Check sheet for the modelled part. Datum: model origin and axes. Units: mm. A direction names the side the tool comes from. Give positions to 0.01 mm unless a question says otherwise; leave off trailing zeros. Loops run counter-clockwise (first coordinate to the right, second up) from the corner with the lowest first, then second, coordinate; pieces in that order, holes last. Notation, with made-up numbers: (74, -4.75) -> (84, -4.75) arc R11 cw to (84, 11.25) -> close; hole circle Ø7 at (8.25, -18.75). An arc over 180 degrees is marked (long way). Write each question's results on one line, items separated by ' | '. Start each with the question number.
1. Material ranges on L1, parallel to Y at x = -53, z = -9; L2, parallel to X at y = 81, z = -19; L3, parallel to Z at x = 54.1, y = 90, recorded low to high. Write a range as from..to.
2. Gauge pin test, flat ends, axial feed: pin 1 Ø3 at (y, z) = (142, -9) entering from +X; pin 2 Ø4 at (y, z) = (109.5, 14.5) entering from +X; pin 3 Ø12 at (y, z) = (91, 3.5) entering from -X; pin 4 Ø8 at (x, z) = (-12, -25) entering from +Y. Record the tip position at first contact, or that the pin passes through.
3. Cross-section at D-D on x = -27.5. Record the boundary of the cut face in (y, z), and give its area (3 significant figures).
4. Mould release check, pull along X, two halves, no side actions. Record for faces 1 (the face through (54.54, 143.66, 8.63)), 2 (the face through (19.879, 81.521, 21.747)): +X half, -X half, draft (parallel to the pull), parting line (faces both ways), or undercut.
5. Cross-section at C-C on y = 133.75. Record the boundary of the cut face in (x, z).
6. Tool access check on faces 3 (the face through (-78.5, 100, -25)), 4 (the face through (-54.535, 138.186, 2.307)), 5 (the face through (-81, 100, 19)). Record the directions out of +Z, -Z, +X, -X, +Y, -Y that give a thin tool (end or side, any length) a straight path to the whole face; none if there is none.
7. Cross-section at B-B on x = 67.75. Record the boundary of the cut face in (y, z), and give its area (3 significant figures).
8. Cross-section at A-A on y = 142. Record the boundary of the cut face in (x, z), and give its area (3 significant figures).
from build123d import *

# Parameters (mm, degrees)
SKETCH1_W                 = 75
SKETCH1_H                 = 40
SKETCH1_R                 = 5
SKETCH1_R_2               = 1.7
SKETCH1_W_2               = 10
SKETCH1_H_2               = 20
BOSS_EXTRUDE1_DEPTH       = 3
CUT_EXTRUDE1_DEPTH        = 43.605750786
CUT_EXTRUDE1_DEPTH_BACK   = 43.605750786
SKETCH2_W                 = 67
SKETCH2_H                 = 28
BOSS_EXTRUDE3_DEPTH       = 110
BOSS_EXTRUDE3_DEPTH_BACK  = 3
SKETCH6_W                 = 67
SKETCH6_H                 = 11
CUT_EXTRUDE4_DEPTH        = 122.372360939
SKETCH7_W                 = 70
SKETCH7_H                 = 37
BOSS_EXTRUDE4_DEPTH       = 45
SKETCH8_W                 = 45
SKETCH8_H                 = 62
CUT_EXTRUDE6_DEPTH        = 29
SKETCH11_W                = 45
SKETCH11_H                = 4
CUT_EXTRUDE9_DEPTH        = 157.445677473
SKETCH9_W                 = 38
SKETCH9_H                 = 28.5
CUT_EXTRUDE10_DEPTH       = 204.024629048
SKETCH13_W                = 5
SKETCH13_H                = 38
BOSS_EXTRUDE5_DEPTH       = 32
SKETCH14_R                = 5
SKETCH14_R_2              = 1.7
CUT_EXTRUDE11_DEPTH       = 32
SKETCH15_W                = 165
SKETCH15_H                = 70
SKETCH15_W_2              = 157
SKETCH15_H_2              = 62
BOSS_EXTRUDE6_DEPTH       = 3
SKETCH16_W                = 20
SKETCH16_H                = 4.820648258
CUT_EXTRUDE12_DEPTH       = 159.626132778
SKETCH18_R                = 5
CUT_EXTRUDE14_DEPTH       = 159.626132778
MIRROR6_COPY_1_SKETCH_W   = 5
MIRROR6_COPY_1_SKETCH_H   = 38
MIRROR6_COPY_1_DEPTH      = 32
MIRROR6_COPY_2_SKETCH_R   = 5
MIRROR6_COPY_2_SKETCH_R_2 = 1.7
MIRROR6_COPY_2_DEPTH      = 32
SKETCH19_W                = 38
SKETCH19_H                = 3.5
CUT_EXTRUDE15_DEPTH       = 10
SKETCH20_R                = 1.2
CUT_EXTRUDE16_DEPTH       = 10
SKETCH21_W                = 10
SKETCH21_H                = 80
CUT_EXTRUDE17_DEPTH       = 184.330984833
SKETCH22_W                = 55
SKETCH22_H                = 80
CUT_EXTRUDE18_DEPTH       = 184.330984833
SKETCH23_W                = 67
SKETCH23_H                = 62
BOSS_EXTRUDE7_DEPTH       = 3
SKETCH24_R                = 10
SKETCH24_R_2              = 2.75
CUT_EXTRUDE19_DEPTH       = 111.707949127


with BuildPart() as part:
    # Sketch1 → Boss-Extrude1 (new body)
    with BuildSketch(Plane(origin=(0, 0, 0), x_dir=(1, 0, 0), z_dir=(0, 1, 0))):
        Rectangle(SKETCH1_W, SKETCH1_H)
        with Locations(Location((-21, 0, 0), (0, 0, 270))):
            Circle(SKETCH1_R, mode=Mode.SUBTRACT)
        with Locations(Location((-30, 8.25, 0), (0, 0, 270))):
            Circle(SKETCH1_R_2, mode=Mode.SUBTRACT)
        with Locations(Location((-12, 8.25, 0), (0, 0, 270))):
            Circle(SKETCH1_R_2, mode=Mode.SUBTRACT)
        with Locations(Location((-12, -8.25, 0), (0, 0, 270))):
            Circle(SKETCH1_R_2, mode=Mode.SUBTRACT)
        with Locations(Location((-30, -8.25, 0), (0, 0, 270))):
            Circle(SKETCH1_R_2, mode=Mode.SUBTRACT)
        with Locations(Location((12, 8.25, 0), (0, 0, 90))):
            Circle(SKETCH1_R_2, mode=Mode.SUBTRACT)
        with Locations(Location((12, -8.25, 0), (0, 0, 90))):
            Circle(SKETCH1_R_2, mode=Mode.SUBTRACT)
        with Locations(Location((21, 0, 0), (0, 0, 90))):
            Circle(SKETCH1_R, mode=Mode.SUBTRACT)
        with Locations(Location((30, -8.25, 0), (0, 0, 90))):
            Circle(SKETCH1_R_2, mode=Mode.SUBTRACT)
        with Locations(Location((30, 8.25, 0), (0, 0, 90))):
            Circle(SKETCH1_R_2, mode=Mode.SUBTRACT)
        Rectangle(SKETCH1_W_2, SKETCH1_H_2, mode=Mode.SUBTRACT)
    extrude(amount=BOSS_EXTRUDE1_DEPTH)

    # Sketch2 → Cut-Extrude1 (cut, two sides: drawn at the far end of the back side and taken through both)
    with BuildSketch(Plane(origin=(0, 3, 0), x_dir=(1, 0, 0), z_dir=(0, 1, 0)).offset(-CUT_EXTRUDE1_DEPTH_BACK)):
        Rectangle(SKETCH2_W, SKETCH2_H)
    extrude(amount=CUT_EXTRUDE1_DEPTH + CUT_EXTRUDE1_DEPTH_BACK, mode=Mode.SUBTRACT)

    # Sketch3 → Boss-Extrude3 (add, two sides: drawn at the far end of the back side and taken through both)
    with BuildSketch(Plane(origin=(0, 3, 0), x_dir=(1, 0, 0), z_dir=(0, 1, 0)).offset(-BOSS_EXTRUDE3_DEPTH_BACK)):
        Polygon((37.5, -35), (37.5, -20), (33.5, -20), (-33.5, -20), (-37.5, -20), (-37.5, -35), align=None)
        Polygon((33.5, 20), (37.5, 20), (37.5, 35), (-37.5, 35), (-37.5, 20), (-33.5, 20), align=None)
        Polygon((37.5, -20), (37.5, 20), (33.5, 20), (33.5, 14), (33.5, -14), (33.5, -20), align=None)
        Polygon((-33.5, 14), (-33.5, 20), (-37.5, 20), (-37.5, -20), (-33.5, -20), (-33.5, -14), align=None)
    extrude(amount=BOSS_EXTRUDE3_DEPTH + BOSS_EXTRUDE3_DEPTH_BACK)

    # Sketch6 → Cut-Extrude4 (cut, through all)
    with BuildSketch(Plane(origin=(0, 3, 0), x_dir=(1, 0, 0), z_dir=(0, 1, 0))):
        with Locations((0, -25.5)):
            Rectangle(SKETCH6_W, SKETCH6_H)
        with Locations((0, 25.5)):
            Rectangle(SKETCH6_W, SKETCH6_H)
    extrude(amount=CUT_EXTRUDE4_DEPTH, mode=Mode.SUBTRACT)

    # Sketch7 → Boss-Extrude4 (add)
    with BuildSketch(Plane.ZY.offset(37.5)):
        with Locations((0, 94.5)):
            Rectangle(SKETCH7_W, SKETCH7_H)
    boss_extrude4 = extrude(amount=BOSS_EXTRUDE4_DEPTH)

    # Mirror2: Boss-Extrude4 across plane
    add(boss_extrude4.mirror(Plane(origin=(0, 0, 0), x_dir=(0, 0, 1), z_dir=(1, 0, 0))))

    # Sketch8 → Cut-Extrude6 (cut)
    with BuildSketch(Plane(origin=(0, 113, 0), x_dir=(1, 0, 0), z_dir=(0, 1, 0))):
        with Locations((-56, 0)):
            Rectangle(SKETCH8_W, SKETCH8_H)
        with Locations((56, 0)):
            Rectangle(SKETCH8_W, SKETCH8_H)
    extrude(amount=-CUT_EXTRUDE6_DEPTH, mode=Mode.SUBTRACT)

    # Sketch11 → Cut-Extrude9 (cut, through all)
    with BuildSketch(Plane.XY.offset(35)):
        with Locations((-60, 78)):
            Rectangle(SKETCH11_W, SKETCH11_H)
        with Locations((60, 78)):
            Rectangle(SKETCH11_W, SKETCH11_H)
    extrude(amount=-CUT_EXTRUDE9_DEPTH, mode=Mode.SUBTRACT)

    # Sketch9 → Cut-Extrude10 (cut, through all)
    with BuildSketch(Plane.ZY.offset(82.5)):
        with Locations((0, 98.25)):
            Rectangle(SKETCH9_W, SKETCH9_H)
    extrude(amount=-CUT_EXTRUDE10_DEPTH, mode=Mode.SUBTRACT)

    # Sketch13 → Boss-Extrude5 (add)
    with BuildSketch(Plane(origin=(0, 84, 0), x_dir=(1, 0, 0), z_dir=(0, 1, 0))):
        with Locations((-54.5, 0)):
            Rectangle(SKETCH13_W, SKETCH13_H)
    boss_extrude5 = extrude(amount=BOSS_EXTRUDE5_DEPTH)

    # Sketch14 → Cut-Extrude11 (cut)
    with BuildSketch(Plane.ZY.offset(57)):
        with Locations((0, 98.25)):
            Circle(SKETCH14_R)
        with Locations((-9, 106.5)):
            Circle(SKETCH14_R_2)
        with Locations((9, 106.5)):
            Circle(SKETCH14_R_2)
        with Locations((9, 90)):
            Circle(SKETCH14_R_2)
        with Locations((-9, 90)):
            Circle(SKETCH14_R_2)
    cut_extrude11 = extrude(amount=-CUT_EXTRUDE11_DEPTH, mode=Mode.SUBTRACT)

    # Mirror4: Boss-Extrude5, Cut-Extrude11 across plane
    add(boss_extrude5.mirror(Plane(origin=(0, 0, 0), x_dir=(0, 0, 1), z_dir=(1, 0, 0))))
    add(cut_extrude11.mirror(Plane(origin=(0, 0, 0), x_dir=(0, 0, 1), z_dir=(1, 0, 0))), mode=Mode.SUBTRACT)

    # Sketch15 → Boss-Extrude6 (add)
    with BuildSketch(Plane(origin=(0, 113, 0), x_dir=(1, 0, 0), z_dir=(0, 1, 0))):
        Rectangle(SKETCH15_W, SKETCH15_H)
        Rectangle(SKETCH15_W_2, SKETCH15_H_2, mode=Mode.SUBTRACT)
    extrude(amount=BOSS_EXTRUDE6_DEPTH)

    # Sketch16 → Cut-Extrude12 (cut, through all)
    with BuildSketch(Plane.XY.offset(35)):
        with Locations((0, 11.636111214)):
            Rectangle(SKETCH16_W, SKETCH16_H)
    extrude(amount=-CUT_EXTRUDE12_DEPTH, mode=Mode.SUBTRACT)

    # Sketch18 → Cut-Extrude14 (cut, through all)
    with BuildSketch(Plane.XY.offset(35)):
        with Locations((67.75, 100)):
            Circle(SKETCH18_R)
    cut_extrude14 = extrude(amount=-CUT_EXTRUDE14_DEPTH, mode=Mode.SUBTRACT)

    # Mirror5: Cut-Extrude14 across plane
    add(cut_extrude14.mirror(Plane(origin=(0, 0, 0), x_dir=(0, 0, 1), z_dir=(1, 0, 0))), mode=Mode.SUBTRACT)

    # Mirror6: Boss-Extrude5, Cut-Extrude11 across plane
    add(boss_extrude5.mirror(Plane.ZX.offset(116)))
    add(cut_extrude11.mirror(Plane.ZX.offset(116)), mode=Mode.SUBTRACT)

    # Mirror6 copy 1 sketch → Mirror6 copy 1 (add)
    with BuildSketch(Plane(origin=(0, 148, 0), x_dir=(-1, 0, 0), z_dir=(0, -1, 0))):
        with Locations((-54.5, 0)):
            Rectangle(MIRROR6_COPY_1_SKETCH_W, MIRROR6_COPY_1_SKETCH_H)
    extrude(amount=MIRROR6_COPY_1_DEPTH)

    # Mirror6 copy 2 sketch → Mirror6 copy 2 (cut)
    with BuildSketch(Plane(origin=(57, 232, 0), x_dir=(0, 0, 1), z_dir=(1, 0, 0))):
        with Locations((0, 98.25)):
            Circle(MIRROR6_COPY_2_SKETCH_R)
        with Locations((-9, 106.5)):
            Circle(MIRROR6_COPY_2_SKETCH_R_2)
        with Locations((9, 106.5)):
            Circle(MIRROR6_COPY_2_SKETCH_R_2)
        with Locations((9, 90)):
            Circle(MIRROR6_COPY_2_SKETCH_R_2)
        with Locations((-9, 90)):
            Circle(MIRROR6_COPY_2_SKETCH_R_2)
    extrude(amount=-MIRROR6_COPY_2_DEPTH, mode=Mode.SUBTRACT)

    # Sketch19 → Cut-Extrude15 (cut)
    with BuildSketch(Plane(origin=(82.5, 0, 0), x_dir=(0, 0, -1), z_dir=(1, 0, 0))):
        with Locations((0, 114.25)):
            Rectangle(SKETCH19_W, SKETCH19_H)
    cut_extrude15 = extrude(amount=-CUT_EXTRUDE15_DEPTH, mode=Mode.SUBTRACT)

    # Mirror7: Cut-Extrude15 across plane
    add(cut_extrude15.mirror(Plane(origin=(0, 0, 0), x_dir=(0, 0, 1), z_dir=(1, 0, 0))), mode=Mode.SUBTRACT)

    # Sketch20 → Cut-Extrude16 (cut)
    with BuildSketch(Plane(origin=(0, 3, 0), x_dir=(1, 0, 0), z_dir=(0, 1, 0))):
        with Locations(Location((-24, 17.5, 0), (0, 0, 270))):
            Circle(SKETCH20_R)
        with Locations(Location((-12, 17.5, 0), (0, 0, 270))):
            Circle(SKETCH20_R)
        with Locations(Location((12, 17.5, 0), (0, 0, 270))):
            Circle(SKETCH20_R)
        with Locations(Location((-24, -17.5, 0), (0, 0, 270))):
            Circle(SKETCH20_R)
        with Locations(Location((-12, -17.5, 0), (0, 0, 270))):
            Circle(SKETCH20_R)
        with Locations(Location((24, 17.5, 0), (0, 0, 270))):
            Circle(SKETCH20_R)
        with Locations(Location((12, -17.5, 0), (0, 0, 270))):
            Circle(SKETCH20_R)
        with Locations(Location((24, -17.5, 0), (0, 0, 270))):
            Circle(SKETCH20_R)
    extrude(amount=-CUT_EXTRUDE16_DEPTH, mode=Mode.SUBTRACT)

    # Sketch21 → Cut-Extrude17 (cut, through all)
    with BuildSketch(Plane.XY.offset(35)):
        with Locations((32.5, 40)):
            Rectangle(SKETCH21_W, SKETCH21_H)
        with Locations((-32.5, 40)):
            Rectangle(SKETCH21_W, SKETCH21_H)
    extrude(amount=-CUT_EXTRUDE17_DEPTH, mode=Mode.SUBTRACT)

    # Sketch22 → Cut-Extrude18 (cut, through all)
    with BuildSketch(Plane.XY.offset(35)):
        with Locations((0, 40)):
            Rectangle(SKETCH22_W, SKETCH22_H)
    extrude(amount=-CUT_EXTRUDE18_DEPTH, mode=Mode.SUBTRACT)

    # Sketch23 → Boss-Extrude7 (add)
    with BuildSketch(Plane.XZ.offset(-80)):
        Rectangle(SKETCH23_W, SKETCH23_H)
    extrude(amount=-BOSS_EXTRUDE7_DEPTH)

    # Sketch24 → Cut-Extrude19 (cut, through all)
    with BuildSketch(Plane(origin=(0, 83, 0), x_dir=(1, 0, 0), z_dir=(0, 1, 0))):
        with Locations(Location((0, 0, 0), (0, 0, 270))):
            Circle(SKETCH24_R)
        with Locations(Location((-20, 19, 0), (0, 0, 270))):
            Circle(SKETCH24_R_2)
        with Locations(Location((-20, -19, 0), (0, 0, 270))):
            Circle(SKETCH24_R_2)
        with Locations(Location((20, -19, 0), (0, 0, 90))):
            Circle(SKETCH24_R_2)
        with Locations(Location((20, 19, 0), (0, 0, 90))):
            Circle(SKETCH24_R_2)
    extrude(amount=-CUT_EXTRUDE19_DEPTH, mode=Mode.SUBTRACT)


solid = part.part
Geometry says:
1) L1: 80..88.3, 91.7..104.8, 108.2..123.8, 127.2..140.3, 143.7..148 | L2: -82.5..-22.75, -17.25..17.25, 22.75..82.5 | L3: -35..-31, -19..-10.7, -7.3..7.3, 10.7..19, 31..35
2) pin 1: through | pin 2: x = 57 | pin 3: x = -57 | pin 4: y = 83
3) outline: (80, -35) -> (116, -35) -> (116, -31) -> (83, -31) -> (83, 31) -> (116, 31) -> (116, 35) -> (80, 35) -> close | area: 474 mm^2
4) face 1: draft | face 2: undercut
5) outline: (-57, -19) -> (-52, -19) -> (-52, -5) -> (-57, -5) -> close; (-57, 5) -> (-52, 5) -> (-52, 19) -> (-57, 19) -> close; (52, -19) -> (57, -19) -> (57, -5) -> (52, -5) -> close; (52, 5) -> (57, 5) -> (57, 19) -> (52, 19) -> close
6) face 3: +Y | face 4: +X, -X | face 5: -X, +Y
7) outline: (80, -35) -> (95, -35) -> (95, -31) -> (84, -31) -> (84, 31) -> (95, 31) -> (95, 35) -> (80, 35) -> close; (105, -35) -> (116, -35) -> (116, -31) -> (105, -31) -> close; (105, 31) -> (116, 31) -> (116, 35) -> (105, 35) -> close | area: 456 mm^2
8) outline: (-57, -19) -> (-52, -19) -> (-52, -10.7) -> (-57, -10.7) -> close; (-57, -7.3) -> (-52, -7.3) -> (-52, 7.3) -> (-57, 7.3) -> close; (-57, 10.7) -> (-52, 10.7) -> (-52, 19) -> (-57, 19) -> close; (52, -19) -> (57, -19) -> (57, -10.7) -> (52, -10.7) -> close; (52, -7.3) -> (57, -7.3) -> (57, 7.3) -> (52, 7.3) -> close; (52, 10.7) -> (57, 10.7) -> (57, 19) -> (52, 19) -> close | area: 312 mm^2
